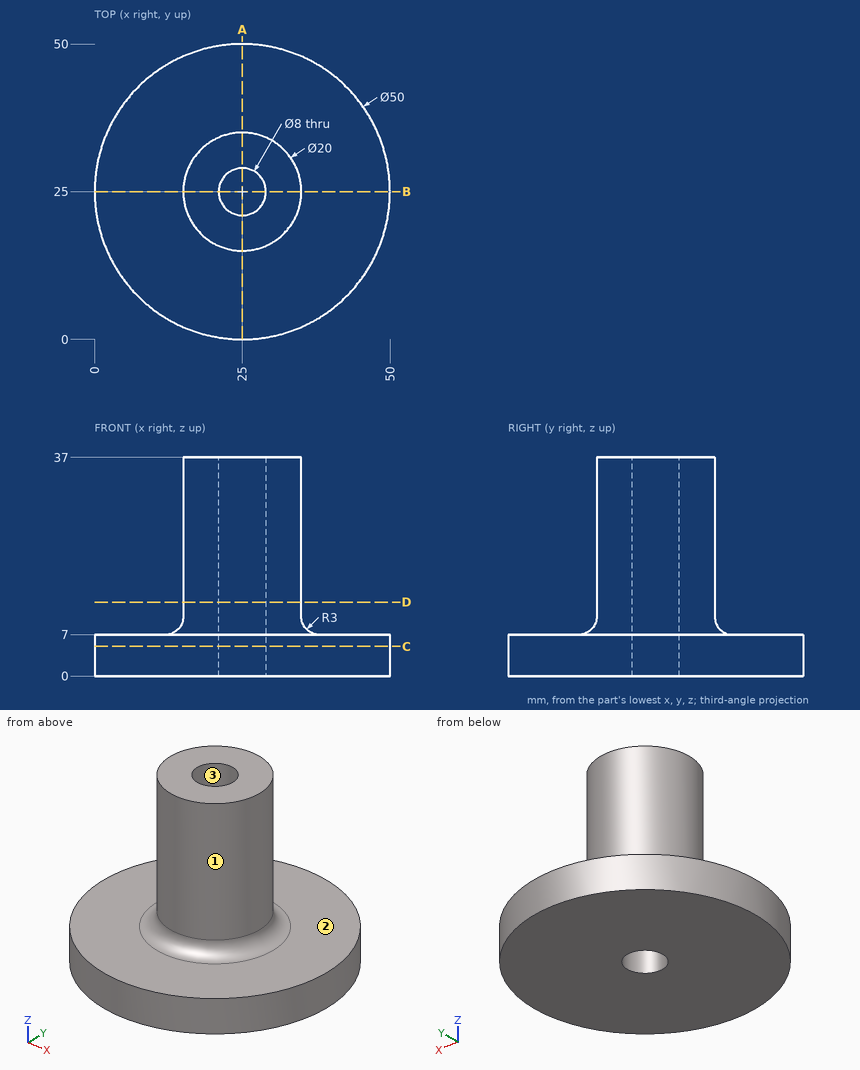
Could you check a few things on this drawing? It's one solid part, dimensions in mm from its lowest x, y, z. Round coordinates to 2 decimals unless told otherwise and drop trailing zeros. Order: outer loops, then holes, each group sorted by start corner. A loop starts at its lowest first (then second) coordinate and runs counter-clockwise, first axis right, second up.
(1) I'm going to push flat-ended pins straight in: pin 1 (6 mm diameter, centred on x = 26.5, y = 16.5, fed in from -Z); pin 2 (4 mm diameter, centred on x = 34.5, z = 32, fed in from -Y); pin 3 (8 mm diameter, centred on x = 39, y = 9, fed in from +Z); pin 4 (10 mm diameter, centred on x = 6, z = 32.5, fed in from -Y). Where does each tip first touch, or does it pass through?
Response values:
pin 1: stops at z = 0
pin 2: stops at y = 18.39
pin 3: stops at z = 7
pin 4: passes through
(2) Imagine slicing it at D-D (z = 12.5). Write out the boundary of the cut face in (x, y), plus the area to 3 significant figures.
Response values:
outline: circle Ø20 at (25, 25); hole circle Ø8 at (25, 25)
area: 264 mm2
(3) Please list where these lines run through material, in increasing order: line 1 along Y through (x, z) = (25, 28); line 2 along Z through (x, y) = (17, 47.5); line 3 along Y through (x, z) = (27.5, 20.5).
Response values:
line 1: y = 15 to 21, 29 to 35
line 2: z = 0 to 7
line 3: y = 15.32 to 21.88, 28.12 to 34.68
(4) If we mould it in two halves opening along X, with no side actions, what happens to the marked faces 1, 2 and 3? For each: released by +X, released by -X, zero draft, split by the parting line, or undercut.
Response values:
face 1: split by the parting line
face 2: zero draft
face 3: undercut
(5) Imagine slicing it at A-A (x = 25). Write out the boundary of the cut face in (y, z).
Response values:
outline: (0, 0) - (21, 0) - (21, 37) - (15, 37) - (15, 10) arc R3 cw to (12, 7) - (0, 7) - close; (29, 0) - (50, 0) - (50, 7) - (38, 7) arc R3 cw to (35, 10) - (35, 37) - (29, 37) - close
(6) Imagine slicing it at C-C (z = 5). Write out the boundary of the cut face in (x, y), plus the area to 3 significant figures.
Response values:
outline: circle Ø50 at (25, 25); hole circle Ø8 at (25, 25)
area: 1,910 mm2
